The listing builds one solid part. Answer for the finished solid, in the listing's coordinates (mm). Face numbers are marked on the shaded views. A direction names the side the tool comes from. Give positions to 0.01 mm unless a question says otherwise; leave off trailing zeros. Loops run counter-clockwise (first coordinate to the right, second up) from the corner with the lowest first, then second, coordinate; pieces in that order, holes last. Notation, with made-up numbers: M 27.25,85.5 L 41.25,85.5 A26 ccw 41.25,108.5 Z; hole C 70.25,44.5 d3. An arc over 180 degrees is marked long. One line per item, written item: value. Start each with the question number.
Q1. A cutting plane is placed at D-D, the plane y = -34. Determine the outline of the cut face in (x, z), and give its area (3 significant figures).
Q2. Consider L1, parallel to Y at x = 0, z = 24; L2, parallel to Z at x = 58, y = -19; L3, parallel to X at y = -60.5, z = 23.5. Determine where each line is inside the solid, lowest interval first.
Q3. A cutting plane is placed at A-A, the plane z = 8.5. Determine the outline of the cut face in (x, y).
Q4. Flat-ended cylindrical pins translate along their axes: pin 1 (1 mm diameter, centred on y = -3.5, z = 3.5, fed in from -X); pin 2 (1.5 mm diameter, centred on y = -58.5, z = 13.5, fed in from -X); pin 3 (20.5 mm diameter, centred on x = 37.19, y = -12.02, fed in from -Z); pin 4 (3 mm diameter, centred on y = -55, z = 13.5, fed in from -X). Find the tip coordinate at first contact, or state that the pin passes through.
Q5. For the marked faces 1 and 2, determine the directions among +Z, -Z, +X, -X, +Y, -Y from which every point of the face is accessible in a straight line to the end or side of a thin tool.
Q6. A cutting plane is placed at B-B, the plane y = -14. Determine the outline of the cut face in (x, z), and give its area (3 significant figures).
Q7. The mould has two halves that part along Y. Classify the marked faces 3, 4 and 5: +Y half, -Y half, draft (parallel to the pull), parting line (faces both ways), or undercut.
Q8. A cutting plane is placed at C-C, the plane x = 40.5. Determine the outline of the cut face in (y, z), and give its area (3 significant figures).
from build123d import *

# Parameters (mm, degrees)
F1_DEPTH = 25.4
F2_T     = -0.762
F3_R     = 12.012936
F4_DEPTH = 25.4
F5_R     = 12.868017
F5_R_2   = 9.8367
F6_DEPTH = 25.4


with BuildPart() as f1:
    # F0 (on Top) → F1 (new body)
    with BuildSketch(Plane.XY):
        Polygon((37.931472, 17.940195), (-39.611701, 17.940195), (-75.17679, -9.851208), (0, -73.559731), (73.252261, -9.331114), align=None)
    extrude(amount=F1_DEPTH)

    # F2
    f2_openings = [f1.faces().sort_by_distance(p)[0] for p in [
        (-0.795151, -17.594404, 25.4),
    ]]
    offset(amount=F2_T, openings=f2_openings)

    # F3 (on face) → F4 (cut)
    with BuildSketch(Plane(origin=(0, 0, 0), x_dir=(1, 0, 0), z_dir=(0, 0, -1))):
        with Locations((0, 27.955376)):
            Circle(F3_R)
    extrude(amount=-F4_DEPTH, mode=Mode.SUBTRACT)

    # F5 (on face) → F6 (cut)
    with BuildSketch(Plane(origin=(0, 0, 0), x_dir=(1, 0, 0), z_dir=(0, 0, -1))):
        with Locations((37.186667, 12.019401)):
            Circle(F5_R)
        with Locations((-27.019626, 6.043865)):
            Circle(F5_R_2)
    extrude(amount=-F6_DEPTH, mode=Mode.SUBTRACT)


solid = f1.part
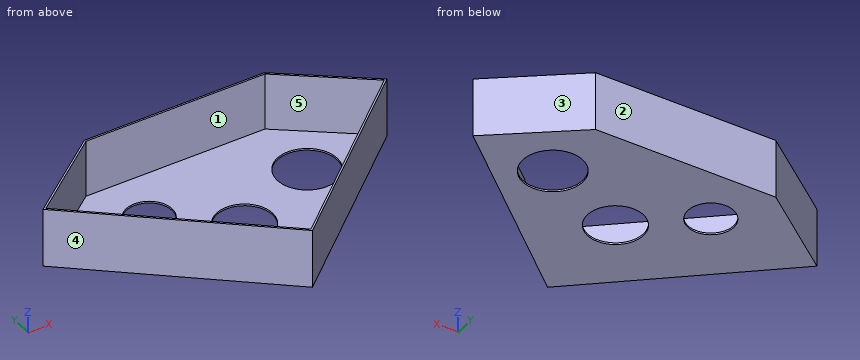
Answer block:
1. outline: M -46.68,0 L -10.38,0 L -10.38,0.76 L -45.5,0.76 L -45.5,25.4 L -46.68,25.4 Z; M 10.38,0 L 45.12,0 L 45.12,25.4 L 43.96,25.4 L 43.96,0.76 L 10.38,0.76 Z
1. area: 112 mm^2
2. L1: -73.56 to -72.55, 17.18 to 17.94
2. L2: 0 to 0.76
2. L3: -15.41 to -14.23, 13.74 to 14.89
3. outline: M -75.18,-9.85 L 0,-73.56 L 73.25,-9.33 L 37.93,17.94 L -39.61,17.94 Z; hole M -73.97,-9.88 L -0.01,-72.55 L 72.05,-9.37 L 37.67,17.18 L -39.35,17.18 Z
4. pin 1: x = -67.69
4. pin 2: x = -18.66
4. pin 3: through
4. pin 4: x = -23.67
5. face 1: +Z
5. face 2: +Z, -Z, +X, -X, +Y
6. outline: M -70.28,0 L -32.8,0 L -32.8,0.76 L -69.1,0.76 L -69.1,25.4 L -70.28,25.4 Z; M -21.24,0 L 24.47,0 L 24.47,0.76 L -21.24,0.76 Z; M 49.9,0 L 67.93,0 L 67.93,25.4 L 66.77,25.4 L 66.77,0.76 L 49.9,0.76 Z
6. area: 135 mm^2
7. face 3: +Y half
7. face 4: -Y half
7. face 5: undercut
8. outline: M -38.05,0 L -24.45,0 L -24.45,0.76 L -37.04,0.76 L -37.04,25.4 L -38.05,25.4 Z; M 0.41,0 L 15.96,0 L 15.96,25.4 L 14.99,25.4 L 14.99,0.76 L 0.41,0.76 Z
8. area: 70.9 mm^2
